Answer from the drawing. Dimensions are ordinates in mm from the lowest x, y and z of the part. A direction names the side the tool comes from. Coordinates: 2 decimals unless noted, no trailing zeros. Order: outer loops, then holes, each group sorted by start corner. A loop starts at its lowest first (then second) coordinate and runs counter-clockwise, first axis right, second up. Notation, with made-up numbers: M 26.5,-24.75 L 47.5,-24.75 A25 cw 47.5,-11.75 Z; hole C 50.25,38 d3. An arc over 180 degrees is marked long. Write each question's results on one line, items separated by ' | '.
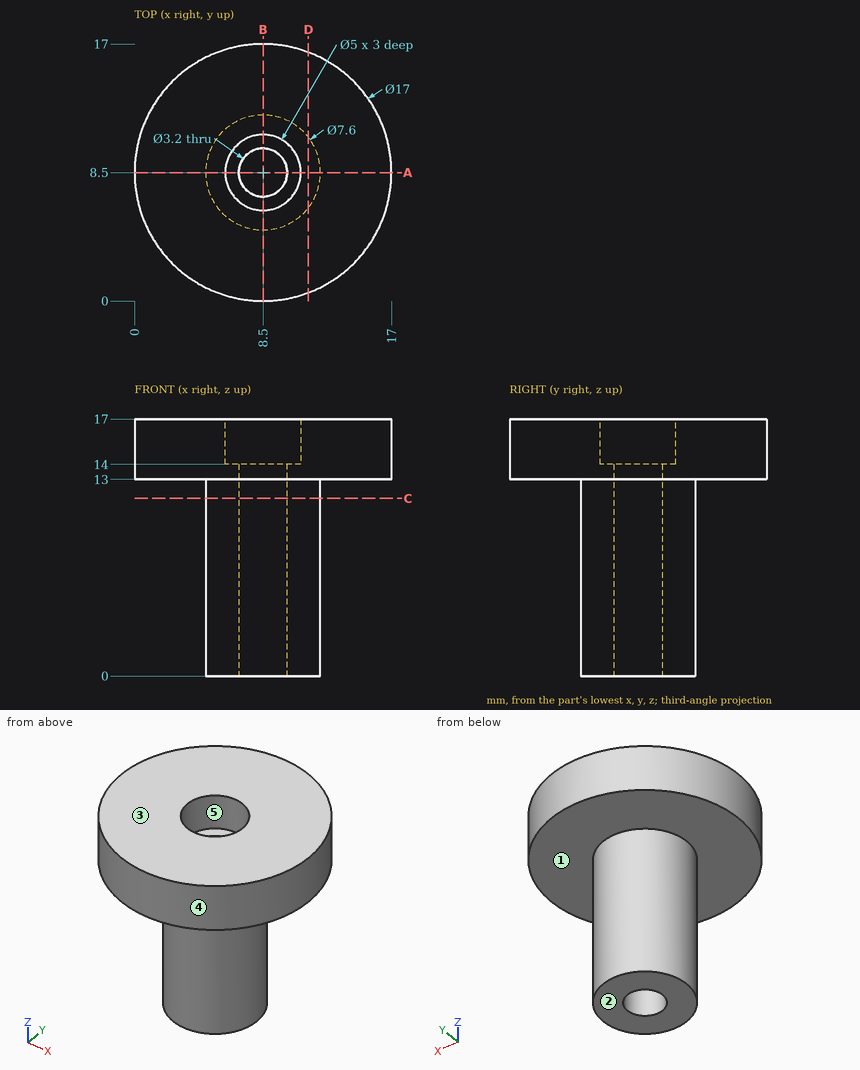
(1) Straight lines are drawn through the part: line 1 (Y direction, x = 8.5, z = 9.5); line 2 (Y direction, x = 8.5, z = 15.85); line 3 (Z direction, x = 8.25, y = 3.25). For each, find the intervals that lie inside material, in ascending order.
Conclusion:
line 1: 4.7 to 6.9, 10.1 to 12.3 | line 2: 0 to 6, 11 to 17 | line 3: 13 to 17
(2) Given pin 1 (4 mm diameter, centred on x = 8.5, y = 8.5, fed in from +Z); pin 2 (1 mm diameter, centred on y = 9.5, z = 14, fed in from -X); pin 3 (5 mm diameter, centred on x = 7.5, z = 13.5, fed in from -Y); pin 4 (1 mm diameter, centred on x = 8.5, z = 7, fed in from -Y), each flat-ended and moving along its own axis, determine where each tip first touches the part or whether it passes through.
Conclusion:
pin 1: z = 14 | pin 2: x = 0.01 | pin 3: y = 0 | pin 4: y = 4.7
(3) The part is cut by section D-D, the plane x = 11.5. Write down the section's boundary in (y, z).
Conclusion:
outline: M 0.55,13 L 6.17,13 L 6.17,0 L 10.83,0 L 10.83,13 L 16.45,13 L 16.45,17 L 0.55,17 Z
(4) For the marked faces 1 and 2, determine the directions among +Z, -Z, +X, -X, +Y, -Y from which every point of the face is accessible in a straight line to the end or side of a thin tool.
Conclusion:
face 1: -Z | face 2: -Z, +X, -X, +Y, -Y
(5) The part is cut by section C-C, the plane z = 11.75. Write down the section's boundary in (x, y).
Conclusion:
outline: C 8.5,8.5 d7.6; hole C 8.5,8.5 d3.2
(6) The part is cut by section A-A, the plane y = 8.5. Write down the section's boundary in (x, z).
Conclusion:
outline: M 0,13 L 4.7,13 L 4.7,0 L 6.9,0 L 6.9,14 L 6,14 L 6,17 L 0,17 Z; M 10.1,0 L 12.3,0 L 12.3,13 L 17,13 L 17,17 L 11,17 L 11,14 L 10.1,14 Z
(7) The mould has two halves that part along X. Classify the marked faces 3, 4 and 5: pulls with the +X half, pulls with the -X half, needs draft (parallel to the pull), parting line crosses it, or undercut.
Conclusion:
face 3: needs draft | face 4: parting line crosses it | face 5: undercut
